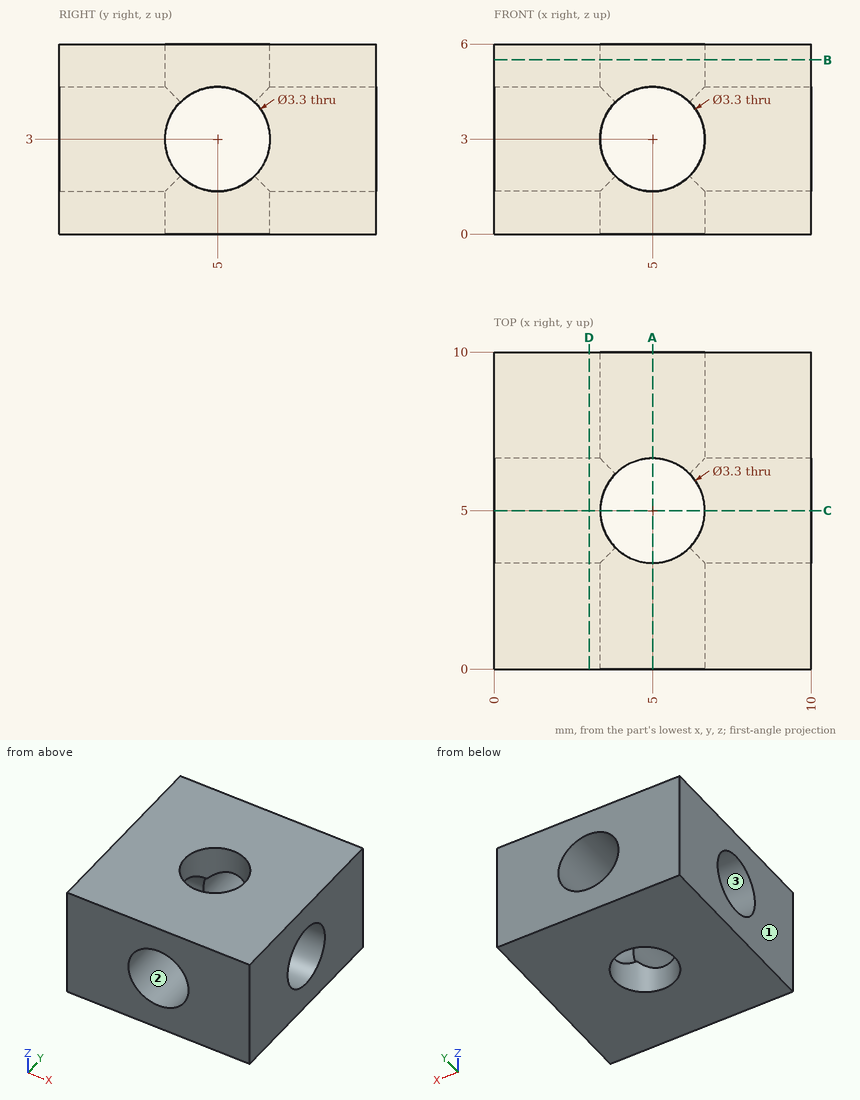
Geometry check sheet. Reference: drawing and pictorial views, mm from the part's lowest x, y, z. Round coordinates to 2 decimals unless told otherwise and drop trailing zeros. Order: outer loops, then holes, each group sorted by start corner. A loop starts at its lowest first (then second) coordinate and runs counter-clockwise, first axis right, second up. Notation, with made-up numbers: M -5.5,52 L 29.5,52 A23 ccw 29.5,88 Z; hole C 87,27 d4. An arc over 180 degrees is marked long. One line per item, written item: value. Start each with the question number.
1. Release check for a two-part mould opening along X. For the marked faces 1, 2 and 3 record: released by +X, released by -X, zero draft, split by the parting line, or undercut.
2. Section check B-B on z = 5.5. Enter the section's corners in (x, y).
3. Scan lines: line 1 along X through (y, z) = (2.85, 3); line 2 along Z through (x, y) = (9, 5). Record each from-to range of solid material in increasing order.
4. Gauge pin test, flat ends, axial feed: P1, Ø1.5, axis at x = 2, y = 9, coming from the -Z side; P2, Ø2, axis at y = 5, z = 3, coming from the -X side. Record the tip position at first contact, or that the pin passes through.
5. Section check A-A on x = 5. Enter the section's corners in (y, z), and give its area (3 significant figures).
6. Section check D-D on x = 3. Enter the section's corners in (y, z), and give its area (3 significant figures).
Results found:
1. face 1: released by -X
1. face 2: undercut
1. face 3: zero draft
2. outline: M 0,0 L 10,0 L 10,10 L 0,10 Z; hole C 5,5 d3.3
3. line 1: 0 to 3.35, 6.65 to 10
3. line 2: 0 to 1.35, 4.65 to 6
4. P1: z = 0
4. P2: through
5. outline: M 0,0 L 3.35,0 L 3.35,1.35 L 0,1.35 Z; M 0,4.65 L 3.35,4.65 L 3.35,6 L 0,6 Z; M 6.65,0 L 10,0 L 10,1.35 L 6.65,1.35 Z; M 6.65,4.65 L 10,4.65 L 10,6 L 6.65,6 Z
5. area: 18.1 mm^2
6. outline: M 0,0 L 10,0 L 10,6 L 0,6 Z; hole C 5,3 d3.3
6. area: 51.4 mm^2
